```python
from build123d import *

# Parameters (mm, degrees)
BOSS_EXTRUDE1_DEPTH           = 4.7625
SKETCH2_R                     = 6.9977
SKETCH2_R_2                   = 1.4986
SKETCH2_R_3                   = 0.9906
SKETCH2_R_4                   = 4.7625
GEARBOX_WITH_PRESS_FITS_DEPTH = 412.602247496
SKETCH6_R                     = 1.59385
CUT_EXTRUDE2_DEPTH            = 412.602247496
F_4_CLEARANCE_HOLE2_D         = 3.2639
F_2_CLEARANCE_HOLE1_D         = 2.4384
F_2_CLEARANCE_HOLE1_DEPTH     = 4.826
F_2_CLEARANCE_HOLE1_TIP       = 0.732569267
F_4_CLEARANCE_HOLE1_D         = 3.2639
F_4_CLEARANCE_HOLE1_DEPTH     = 4.826
F_4_CLEARANCE_HOLE1_TIP       = 0.980574487


with BuildPart() as part:
    # Sketch1 → Boss-Extrude1 (new body)
    with BuildSketch(Plane(origin=(0, 0, 0), x_dir=(0, 0, -1), z_dir=(1, 0, 0))):
        Polygon((33.297595377, -40.64), (312.697595377, -40.64), (345.995190754, -12.7), (409.563327383, 40.64), (312.697595377, 40.64), (33.297595377, 40.64), (0, 12.7), (-63.568136629, -40.64), align=None)
    extrude(amount=BOSS_EXTRUDE1_DEPTH)

    # Sketch2 → Gearbox (with Press fits) (cut, through all)
    with BuildSketch(Plane(origin=(4.7625, 0, 0), x_dir=(0, 0, -1), z_dir=(1, 0, 0))):
        with Locations((300.047997426, 10)):
            Circle(SKETCH2_R)
        with Locations((282.214696722, 8)):
            Circle(SKETCH2_R_2)
        with Locations((270.217776392, 15.933400182)):
            Circle(SKETCH2_R_3)
        with Locations((331.004197426, 10)):
            Circle(SKETCH2_R_4)
    extrude(amount=-GEARBOX_WITH_PRESS_FITS_DEPTH, mode=Mode.SUBTRACT)

    # Sketch6 → Cut-Extrude2 (cut, through all)
    with BuildSketch(Plane(origin=(4.7625, 0, 0), x_dir=(0, 0, -1), z_dir=(1, 0, 0))):
        with Locations((287.297595377, 36.83)):
            Circle(SKETCH6_R)
        with Locations((230.147595377, 36.83)):
            Circle(SKETCH6_R)
        with Locations((172.997595377, 36.83)):
            Circle(SKETCH6_R)
        with Locations((115.847595377, 36.83)):
            Circle(SKETCH6_R)
        with Locations((58.697595377, 36.83)):
            Circle(SKETCH6_R)
        with Locations((58.697595377, -36.83)):
            Circle(SKETCH6_R)
        with Locations((115.847595377, -36.83)):
            Circle(SKETCH6_R)
        with Locations((172.997595377, -36.83)):
            Circle(SKETCH6_R)
        with Locations((230.147595377, -36.83)):
            Circle(SKETCH6_R)
        with Locations((287.297595377, -36.83)):
            Circle(SKETCH6_R)
    extrude(amount=-CUT_EXTRUDE2_DEPTH, mode=Mode.SUBTRACT)

    # #4 Clearance Hole2 (through all)
    with Locations(Plane(origin=(4.7625, 0, 0), x_dir=(0, 0, -1), z_dir=(1, 0, 0))):
        with Locations((147.597595377, 35.56), (198.397595377, 35.56), (198.397595377, -35.56), (147.597595377, -35.56), (147.597595377, 0), (198.397595377, 0)):
            Hole(F_4_CLEARANCE_HOLE2_D / 2)

    # #2 Clearance Hole1
    with Locations(Plane(origin=(4.7625, 0, 0), x_dir=(0, 0, -1), z_dir=(1, 0, 0))):
        with Locations((248.047997486, -3), (248.047997486, 23), (271.047997556, -3), (312.047997486, -3), (279.047997486, 23), (312.047997486, 23)):
            Hole(F_2_CLEARANCE_HOLE1_D / 2, depth=F_2_CLEARANCE_HOLE1_DEPTH)
            with Locations((0, 0, -(F_2_CLEARANCE_HOLE1_DEPTH + F_2_CLEARANCE_HOLE1_TIP / 2))):  # 118° drill point
                Cone(0, F_2_CLEARANCE_HOLE1_D / 2, F_2_CLEARANCE_HOLE1_TIP, mode=Mode.SUBTRACT)

    # #4 Clearance Hole1
    with Locations(Plane(origin=(4.7625, 0, 0), x_dir=(0, 0, -1), z_dir=(1, 0, 0))):
        with Locations((327.962613202, -22.8575274), (342.555759844, -10.612423436), (367.850547356, 10.612423436), (382.443693997, 22.8575274), (-36.448503243, -22.8575274), (-21.855356602, -10.612423436), (3.43943091, 10.612423436), (18.032577552, 22.8575274)):
            Hole(F_4_CLEARANCE_HOLE1_D / 2, depth=F_4_CLEARANCE_HOLE1_DEPTH)
            with Locations((0, 0, -(F_4_CLEARANCE_HOLE1_DEPTH + F_4_CLEARANCE_HOLE1_TIP / 2))):  # 118° drill point
                Cone(0, F_4_CLEARANCE_HOLE1_D / 2, F_4_CLEARANCE_HOLE1_TIP, mode=Mode.SUBTRACT)


solid = part.part
```
Read the model definition and answer for the solid it produces. Units are mm, in the model's axes. Give positions to 0.01 mm unless a question says otherwise; leave off trailing zeros.
Item 1: Each of these flat-tipped pins is pushed along its axis until it touches: pin 1 Ø12 at (y, z) = (4, -354) entering from -X; pin 2 Ø1.9 at (y, z) = (36.83, -173) entering from +X; pin 3 Ø1 at (x, y) = (2.5, 3) entering from +Z. Where does it stop, or does it pass through?
Item 2: The mould has two halves that part along Y. Classify faces 1 (the cylindrical face through (2.415, 11.431, -335.547)), 2 (the flat face through (4.762, 1, -170)): released by +Y, released by -Y, zero draft, split by the parting line, or undercut.
Item 3: The part is cut by section A-A (x = 1). Give the number of separate pieces and of enclosed holes in the cut face, and give its area (3 significant figures).
Item 4: Find the intervals of material crossed by line 1 along Z through (x, y) = (0.4, 13); line 2 along Z through (x, y) = (2.45, 4); line 3 along Z through (x, y) = (0.85, 21), in increasing order.
Taken from the geometry:
1. pin 1: stops at x = 0
1. pin 2: passes through
1. pin 3: stops at z = 12.16
2. face 1: undercut
2. face 2: zero draft
3. separate pieces: 1
3. enclosed holes: 34
3. area: 30,100 mm2
4. line 1: z = -376.62 to -334.7, -327.31 to -306.37, -293.73 to -0.36
4. line 2: z = -365.9 to -303.65, -296.45 to 10.37
4. line 3: z = -386.16 to -9.89
